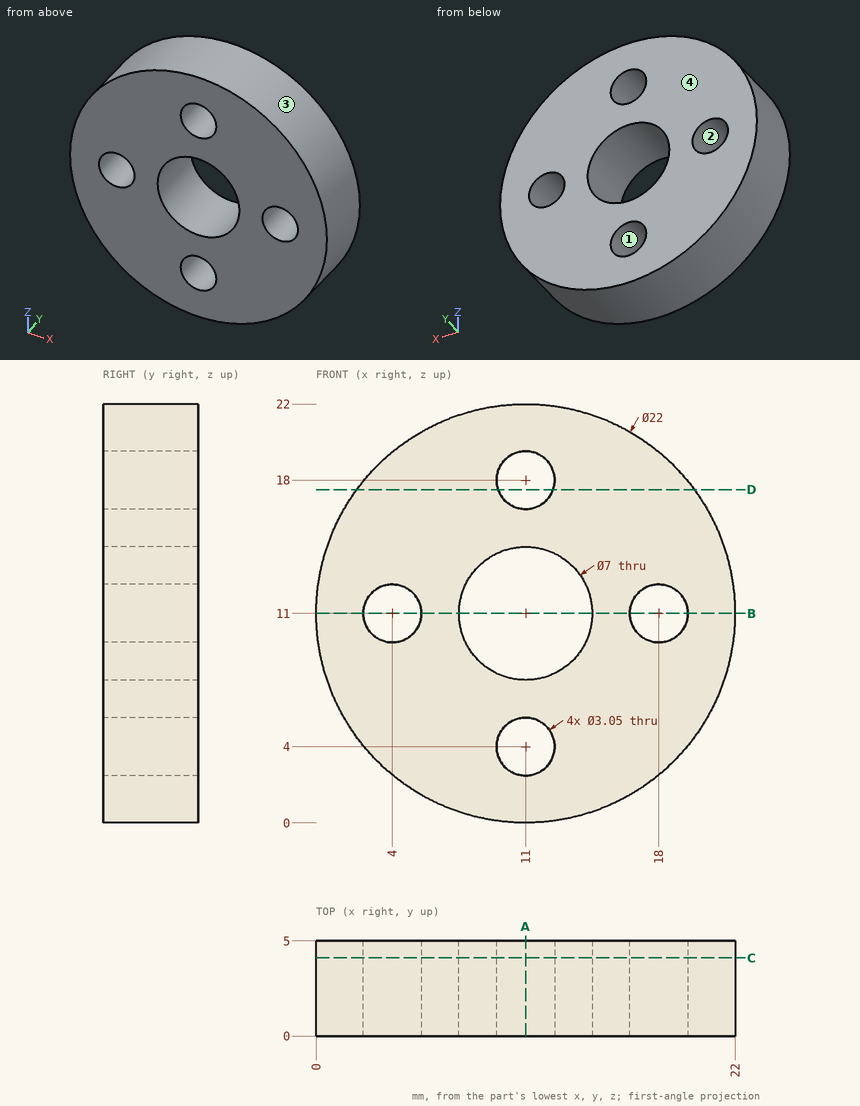
Drawing for the job (mm, zero at the part's lowest x, y, z). Round coordinates to 2 decimals unless told otherwise and drop trailing zeros. Write each loop counter-clockwise with the first axis right and the second up, starting at its lowest first coordinate (ties: lowest second). Pieces come first, ordered by that corner, then holes. Notation, with made-up numbers: (25.5, -27.75) - (48.5, -27.75) arc R15 cw to (48.5, -21.75) - close; hole circle Ø8 at (65.25, -28). An arc over 180 degrees is marked (long way). Return JSON: item names as keys, results as strings. Group by question number.
Item 1: Flat gauge pins, fed straight in: pin 1 Ø2 at (x, y) = (18.5, 4) entering from +Z; pin 2 Ø6.5 at (x, z) = (11, 11) entering from -Y; pin 3 Ø1.5 at (y, z) = (4, 14.5) entering from -X; pin 4 Ø1 at (y, z) = (4, 18) entering from -X. Where does each tip first touch, or does it go through?
Item 2: Band-saw the part on D-D on z = 17.5. List the corners of the cut face in (x, y).
Item 3: Mould opens along Z. For the marked faces 1, 2, 3 and 4 say: +Z half, -Z half, draft (parallel to the pull), parting line (faces both ways), or undercut.
Item 4: Band-saw the part on C-C on y = 4.1. List the corners of the cut face in (x, z) (3 decimals).
Item 5: Probe probe 1 along Z at (x, y) = (11, 1.3) (3 decimals); probe 2 along X at (y, z) = (0.9, 12). List the from-to ranges inside material, lowest first.
Item 6: Band-saw the part on A-A on x = 11. List the corners of the cut face in (y, z) (3 decimals), plus the area to 3 significant figures.
Item 7: Band-saw the part on B-B on z = 11. List the corners of the cut face in (x, y) (3 decimals), plus the area to 3 significant figures.
Resolved:
{
 "1": {"pin 1": "stops at z = 19.87", "pin 2": "passes through", "pin 3": "stops at x = 0.35", "pin 4": "stops at x = 2.13"},
 "2": {"outline": "(2.13, 0) - (9.56, 0) - (9.56, 5) - (2.13, 5) - close; (12.44, 0) - (19.87, 0) - (19.87, 5) - (12.44, 5) - close"},
 "3": {"face 1": "undercut", "face 2": "undercut", "face 3": "parting line", "face 4": "draft"},
 "4": {"outline": "circle Ø22 at (11, 11); hole circle Ø3.05 at (4, 11); hole circle Ø7 at (11, 11); hole circle Ø3.05 at (11, 4); hole circle Ø3.05 at (11, 18); hole circle Ø3.05 at (18, 11)"},
 "5": {"probe 1": "z = 0 to 2.475, 5.525 to 7.5, 14.5 to 16.475, 19.525 to 22", "probe 2": "x = 0.05 to 2.85, 5.15 to 7.65, 14.35 to 16.85, 19.15 to 21.95"},
 "6": {"outline": "(0, 0) - (5, 0) - (5, 2.475) - (0, 2.475) - close; (0, 5.525) - (5, 5.525) - (5, 7.5) - (0, 7.5) - close; (0, 14.5) - (5, 14.5) - (5, 16.475) - (0, 16.475) - close; (0, 19.525) - (5, 19.525) - (5, 22) - (0, 22) - close", "area": "44.5 mm²"},
 "7": {"outline": "(0, 0) - (2.475, 0) - (2.475, 5) - (0, 5) - close; (5.525, 0) - (7.5, 0) - (7.5, 5) - (5.525, 5) - close; (14.5, 0) - (16.475, 0) - (16.475, 5) - (14.5, 5) - close; (19.525, 0) - (22, 0) - (22, 5) - (19.525, 5) - close", "area": "44.5 mm²"}
}
